```python
from build123d import *

# Parameters (mm, degrees)
SKETCH_1_W          = 189.06
SKETCH_1_H          = 44.73
EXTRUDE_1_DEPTH     = 15
CUT_EXTRUDE_4_REACH = 196.858
SKETCH_6_R          = 10
EXTRUDE_2_DEPTH     = 10
SKETCH_7_R          = 1
CUT_EXTRUDE_6_DEPTH = 5
SKETCH_8_R          = 12
SKETCH_8_R_2        = 10
EXTRUDE_3_DEPTH     = 2.5


with BuildPart() as part:
    # 草图1 → 凸台-拉伸1 (new body)
    with BuildSketch(Plane.XY):
        with Locations((94.53, 22.365)):
            Rectangle(SKETCH_1_W, SKETCH_1_H)
    extrude(amount=EXTRUDE_1_DEPTH)

    # 草图4 → 切除-拉伸4 (cut, up to next)
    with BuildSketch(Plane.XY.offset(15), mode=Mode.PRIVATE) as cut_extrude_4_sk1:
        with BuildLine():
            Line((22.27, 44.73), (189.06, 44.73))
            Line((189.06, 44.73), (189.06, 0))
            Line((189.06, 0), (22.27, 0))
            ThreePointArc((22.27, 0), (44.635, 22.365), (22.27, 44.73))
        make_face()
    cut_extrude_4_tool1 = extrude(cut_extrude_4_sk1.sketch, amount=-CUT_EXTRUDE_4_REACH, mode=Mode.PRIVATE) & part.part
    add(cut_extrude_4_tool1.solids().sort_by_distance((114.364224, 22.365, 15))[0], mode=Mode.SUBTRACT)

    # 草图6 → 凸台-拉伸2 (add)
    with BuildSketch(Plane(origin=(0, 0, 0), x_dir=(-1, 0, 0), z_dir=(0, 0, -1))):
        with Locations((-22.27, 22.365)):
            Circle(SKETCH_6_R)
    extrude(amount=EXTRUDE_2_DEPTH)

    # 草图7 → 切除-拉伸6 (cut)
    with BuildSketch(Plane(origin=(0, 0, -10), x_dir=(-1, 0, 0), z_dir=(0, 0, -1))):
        with Locations((-22.27, 29.365)):
            Circle(SKETCH_7_R)
        with Locations((-15.27, -108.576623388)):
            Circle(SKETCH_7_R)
        with Locations((-153.211623388, -115.576623388)):
            Circle(SKETCH_7_R)
        with Locations((-160.211623388, 22.365)):
            Circle(SKETCH_7_R)
    extrude(amount=-CUT_EXTRUDE_6_DEPTH, mode=Mode.SUBTRACT)

    # 草图8 → 凸台-拉伸3 (add)
    with BuildSketch(Plane(origin=(0, 0, 0), x_dir=(-1, 0, 0), z_dir=(0, 0, -1))):
        with Locations((-22.27, 22.365)):
            Circle(SKETCH_8_R)
        with Locations((-22.27, 22.365)):
            Circle(SKETCH_8_R_2, mode=Mode.SUBTRACT)
    extrude(amount=EXTRUDE_3_DEPTH)


solid = part.part
```
The listing builds one solid part. Answer for the finished solid, in the listing's coordinates (mm). A direction names the side the tool comes from. Round coordinates to 2 decimals unless told otherwise and drop trailing zeros. Loops run counter-clockwise (first coordinate to the right, second up) from the corner with the lowest first, then second, coordinate; pieces in that order, holes last.
Q1. Which of the six approach directions +Z, -Z, +X, -X, +Y, -Y give full straight-line access (tool end or side, diameter ignored) to faces 1 (the face through (12, 13, 0)), 2 (the face through (11, 0, 7))?
Q2. For a pull along X with two mould halves and no side action, classify faces 3 (the face through (12.732, 25.369, -6.198)), 4 (the face through (11, 44.73, 7)), 5 (the face through (22, 29, -5)), 6 (the face through (21.316, 29.665, -7.535)) as released by +X, released by -X, zero draft, split by the parting line, or undercut.
Q3. Given pin 1 Ø1 at (x, z) = (6.5, -1.5) entering from +Y; pin 2 Ø0.6 at (x, y) = (22.5, 29.5) entering from -Z; pin 3 Ø4 at (y, z) = (30, -3.5) entering from -X; pin 4 Ø1 at (y, z) = (32, 10.5) entering from +X, each flat-ended and moving along its own axis, determine where each tip first touches the part or whether it passes through.
Q4. Section C-C, the plane z = -6 is taken. Determine the outline of the cut face in (x, y) (3 decimals), then the cut area to 3 significant figures.
Q5. Section B-B, the plane y = 23 is taken. Determine the outline of the cut face in (x, z), then the cut area to 3 significant figures.
Q6. Section D-D, the plane z = 4 is taken. Determine the outline of the cut face in (x, y) (3 decimals), then the cut area to 3 significant figures.
Q7. Section A-A, the plane x = 17.5 is taken. Determine the outline of the cut face in (y, z), then the cut area to 3 significant figures.
Q8. Find the intervals of material crossed by line 1 (Y direction, x = 22.27, z = -8.25) (3 decimals); line 2 (Z direction, x = 12, y = 14.5); line 3 (X direction, y = 22, z = 10.25), in increasing order.
Completed:
1. face 1: -Z
1. face 2: +Z, -Z, +X, -X, -Y
2. face 3: split by the parting line
2. face 4: zero draft
2. face 5: undercut
2. face 6: undercut
3. pin 1: passes through
3. pin 2: stops at z = -5
3. pin 3: stops at x = 11.82
3. pin 4: stops at x = 42.68
4. outline: circle Ø20 at (22.27, 22.365); hole circle Ø2 at (22.27, 29.365)
4. area: 311 mm2
5. outline: (0, 0) - (10.29, 0) - (10.29, -2.5) - (12.29, -2.5) - (12.29, -10) - (32.25, -10) - (32.25, -2.5) - (34.25, -2.5) - (34.25, 0) - (44.63, 0) - (44.63, 15) - (0, 15) - close
5. area: 879 mm2
6. outline: (0, 0) - (22.27, 0) arc R22.365 ccw to (22.27, 44.73) - (0, 44.73) - close
6. area: 1,780 mm2
7. outline: (0, 0) - (11.35, 0) - (11.35, -2.5) - (13.58, -2.5) - (13.58, -10) - (31.15, -10) - (31.15, -2.5) - (33.38, -2.5) - (33.38, 0) - (44.73, 0) - (44.73, 15) - (0, 15) - close
7. area: 858 mm2
8. line 1: y = 12.365 to 28.365, 30.365 to 32.365
8. line 2: z = 0 to 15
8. line 3: x = 0 to 44.63
